Autodesk Inventor part; units mm, degrees
ref_plane "YZ Plane" through (0, 0, 0) normal (1, 0, 0) x (0, 1, 0)
ref_plane "XZ Plane" through (0, 0, 0) normal (0, 1, 0) x (-1, 0, 0)
ref_plane "XY Plane" through (0, 0, 0) normal (0, 0, 1) x (1, 0, 0)
sketch "Sketch1" plane through (0, 0, 0) normal (0, 0, 1) x (1, 0, 0)
  line L0 (0, 31.7899) -> (0, -31.7899)
  line L1 (-70.2899, 0) -> (70.2899, 0)
  line L2 (-49, 22.5) -> (49, 22.5)
  line L3 (50, 21.5) -> (50, -21.5)
  line L4 (-50, -21.5) -> (-50, 21.5)
  line L5 (30, -21.5) -> (30, -20.5)
  line L6 (22, -12.5) -> (-22, -12.5)
  line L7 (-30, -20.5) -> (-30, -21.5)
  arc A0 (-22, -12.5) -> (-30, -20.5) centre (-22, -20.5) ccw
  arc A1 (30, -20.5) -> (22, -12.5) centre (22, -20.5) ccw
  line L8 (49, -22.5) -> (31, -22.5)
  line L9 (-31, -22.5) -> (-49, -22.5)
  arc A2 (-49, 22.5) -> (-50, 21.5) centre (-49, 21.5) ccw
  arc A3 (50, 21.5) -> (49, 22.5) centre (49, 21.5) ccw
  arc A4 (49, -22.5) -> (50, -21.5) centre (49, -21.5) ccw
  arc A5 (30, -21.5) -> (31, -22.5) centre (31, -21.5) ccw
  arc A6 (-31, -22.5) -> (-30, -21.5) centre (-31, -21.5) ccw
  arc A7 (-50, -21.5) -> (-49, -22.5) centre (-49, -21.5) ccw
  point P0 (0, 0)
  point P1 (-50, 22.5)
  point P2 (50, 22.5)
  point P3 (-50, -22.5)
  dimension "d0" = 100
  dimension "d1" = 45
  dimension "d2" = 20
  dimension "d4" = 8
  dimension "d5" = 1
  dimension "d6" = 1
extrude "Extrusion1" add sketch "Sketch1" against normal blind 10
properties part number "SlipersLåda 211018008"
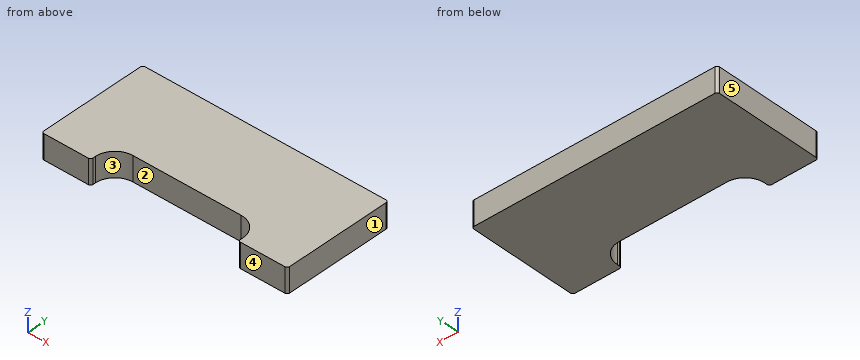
Design review of the part built by this model. Coordinates are the model's own, in mm. Face numbers are marked on the shaded views. A direction names the side the tool comes from. Coordinates: 2 decimals unless noted, no trailing zeros. Loops run counter-clockwise (first coordinate to the right, second up) from the corner with the lowest first, then second, coordinate; pieces in that order, holes last. Notation, with made-up numbers: (86.25, -27.75) - (143.25, -27.75) arc R27 cw to (143.25, 0.25) - close; hole circle Ø9 at (84.25, 21). An arc over 180 degrees is marked (long way). Use CSV: the item, a comma, the result in double quotes. Start each with the question number.
1) Tool access review of the marked faces 1 and 2: name each direction out of +Z, -Z, +X, -X, +Y, -Y from which nothing blocks a thin tool from reaching the whole face with its end or side.
2) Wall thickness on L1, parallel to X at y = -20, z = -7.75; L2, parallel to Y at x = -11.5, z = -5.5; L3, parallel to X at y = -18, z = -9.5: over which ranges is each line inside the solid? List them lowest first. Write a range as from..to.
3) The part is to be moulded in two halves that separate along X. For the marked faces 3, 4 and 5, say which applies: +X half, -X half, draft (parallel to the pull), parting line (faces both ways), or undercut.
4) Consider section C-C on x = -4. Write out the cut boundary in (y, z), then the cut area to 3 significant figures.
5) Consider section A-A on y = -13.5. Write out the cut boundary in (x, z).
6) For pin 1 Ø5 at (x, z) = (-9, -4.5) entering from -Y, flat-tipped, find the tip position at first contact; note if it passes through.
7) Consider section B-B on z = -6.75. Write out the cut boundary in (x, y), then the cut area to 3 significant figures.
Geometry says:
1,face 1,"+Z, -Z, +X, +Y, -Y"
1,face 2,"+Z, -Z, -Y"
2,L1,"-50..-29.98, 29.98..50"
2,L2,"-12.5..22.5"
2,L3,"-50..-29.6, 29.6..50"
3,face 3,"undercut"
3,face 4,"draft"
3,face 5,"-X half"
4,outline,"(-12.5, -10) - (22.5, -10) - (22.5, 0) - (-12.5, 0) - close"
4,area,"350 mm^2"
5,outline,"(-50, -10) - (-25.87, -10) - (-25.87, 0) - (-50, 0) - close; (25.87, -10) - (50, -10) - (50, 0) - (25.87, 0) - close"
6,pin 1,"y = -12.5"
7,outline,"(-50, -21.5) arc R1 ccw to (-49, -22.5) - (-31, -22.5) arc R1 ccw to (-30, -21.5) - (-30, -20.5) arc R8 cw to (-22, -12.5) - (22, -12.5) arc R8 cw to (30, -20.5) - (30, -21.5) arc R1 ccw to (31, -22.5) - (49, -22.5) arc R1 ccw to (50, -21.5) - (50, 21.5) arc R1 ccw to (49, 22.5) - (-49, 22.5) arc R1 ccw to (-50, 21.5) - close"
7,area,"3,930 mm^2"
